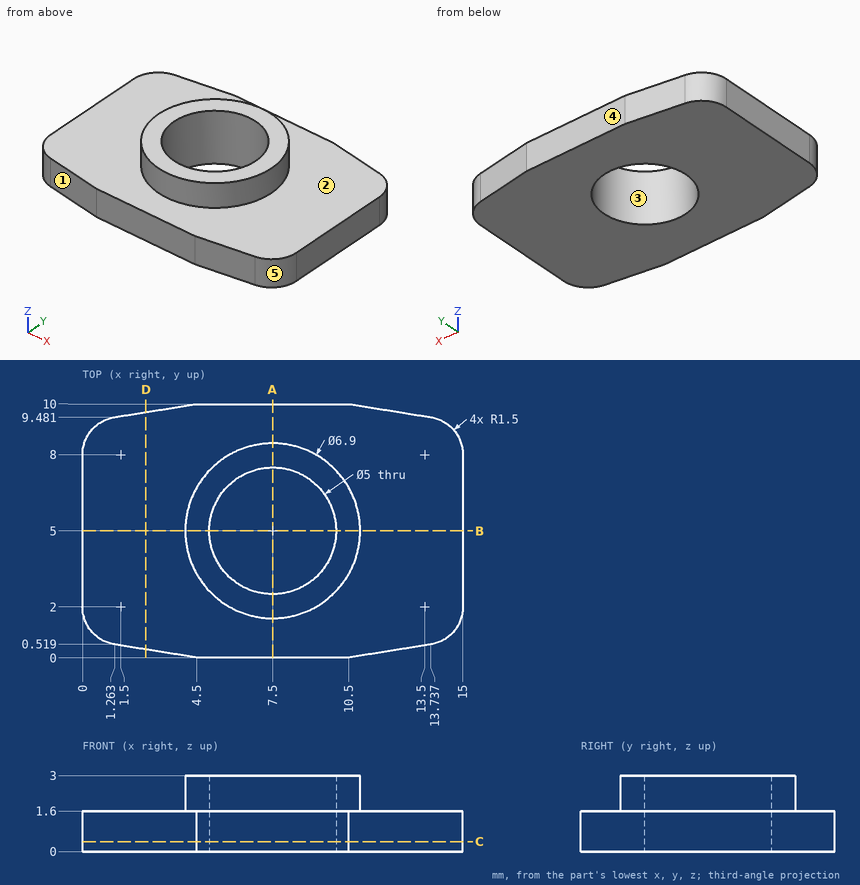
Geometry check sheet. Reference: drawing and pictorial views, mm from the part's lowest x, y, z. A direction names the side the tool comes from. Round coordinates to 2 decimals unless told otherwise and drop trailing zeros. Loops run counter-clockwise (first coordinate to the right, second up) from the corner with the lowest first, then second, coordinate; pieces in that order, holes last.
1. Scan lines: probe 1 along Y at (x, z) = (7.5, 1.8); probe 2 along Y at (x, z) = (7.5, 0.65); probe 3 along Z at (x, y) = (4, 3.75). Record each from-to range of solid material in increasing order.
2. Sectioned sample at D-D on x = 2.5. Record the boundary of the cut face in (y, z).
3. Sectioned sample at A-A on x = 7.5. Record the boundary of the cut face in (y, z).
4. Set-up check for the marked faces 1 and 2: record each of +Z, -Z, +X, -X, +Y, -Y from which the full face is reachable in a straight line by a thin tool's end or side.
5. Sectioned sample at C-C on z = 0.4. Record the boundary of the cut face in (x, y).
6. Sectioned sample at B-B on y = 5. Record the boundary of the cut face in (x, z).
7. Mould release check, pull along X, two halves, no side actions. Record for the marked faces 3, 4 and 5: released by +X, released by -X, zero draft, split by the parting line, or undercut.
Recorded:
1. probe 1: y = 1.55 to 2.5, 7.5 to 8.45
1. probe 2: y = 0 to 2.5, 7.5 to 10
1. probe 3: z = 0 to 1.6
2. outline: (0.32, 0) - (9.68, 0) - (9.68, 1.6) - (0.32, 1.6) - close
3. outline: (0, 0) - (2.5, 0) - (2.5, 3) - (1.55, 3) - (1.55, 1.6) - (0, 1.6) - close; (7.5, 0) - (10, 0) - (10, 1.6) - (8.45, 1.6) - (8.45, 3) - (7.5, 3) - close
4. face 1: +Z, -Z, -X, -Y
4. face 2: +Z
5. outline: (0, 2) arc R1.5 ccw to (1.26, 0.52) - (4.5, 0) - (10.5, 0) - (13.74, 0.52) arc R1.5 ccw to (15, 2) - (15, 8) arc R1.5 ccw to (13.74, 9.48) - (10.5, 10) - (4.5, 10) - (1.26, 9.48) arc R1.5 ccw to (0, 8) - close; hole circle Ø5 at (7.5, 5)
6. outline: (0, 0) - (5, 0) - (5, 3) - (4.05, 3) - (4.05, 1.6) - (0, 1.6) - close; (10, 0) - (15, 0) - (15, 1.6) - (10.95, 1.6) - (10.95, 3) - (10, 3) - close
7. face 3: undercut
7. face 4: zero draft
7. face 5: released by +X
